Build history of the part. All positions in model axes, mm. Give positions to 0.01 mm unless a question says otherwise; leave off trailing zeros. Loops run counter-clockwise (first coordinate to the right, second up) from the corner with the lowest first, then second, coordinate; pieces in that order, holes last. Notation, with made-up numbers: (-3, 17.5) -> (49, 17.5) arc R14 ccw to (49, 34.5) -> close; hole circle Ø4 at (-36, 63). An arc over 180 degrees is marked (long way). Answer in a Markdown table with one row per item. Add a question column.
from build123d import *

# Parameters (mm, degrees)
SKETCH1_W           = 13
SKETCH1_H           = 39
BOSS_EXTRUDE1_DEPTH = 1
SKETCH2_R           = 1.35
CUT_EXTRUDE1_DEPTH  = 2
FILLET1_R           = 1


with BuildPart() as part:
    # Sketch1 → Boss-Extrude1 (new body)
    with BuildSketch(Plane(origin=(0, 0, 0), x_dir=(1, 0, 0), z_dir=(0, 1, 0))):
        Rectangle(SKETCH1_W, SKETCH1_H)
    extrude(amount=BOSS_EXTRUDE1_DEPTH)

    # Sketch2 → Cut-Extrude1 (cut, through all)
    with BuildSketch(Plane(origin=(0, 1, 0), x_dir=(1, 0, 0), z_dir=(0, 1, 0))):
        with Locations((4.5, 0)):
            Circle(SKETCH2_R)
        with Locations((4.5, -17)):
            Circle(SKETCH2_R)
        with Locations((4.5, 17)):
            Circle(SKETCH2_R)
        with Locations((-4.5, 0)):
            Circle(SKETCH2_R)
        with Locations((-4.5, 17)):
            Circle(SKETCH2_R)
        with Locations((-4.5, -17)):
            Circle(SKETCH2_R)
    extrude(amount=-CUT_EXTRUDE1_DEPTH, mode=Mode.SUBTRACT)

    # Fillet1
    fillet1_edges = [part.edges().sort_by_distance(p)[0] for p in [
        (6.5, 0.5, 19.5),
        (-6.5, 0.5, 19.5),
        (-6.5, 0.5, -19.5),
        (6.5, 0.5, -19.5),
    ]]
    fillet(fillet1_edges, radius=FILLET1_R)


solid = part.part
(1) Saw through at B-B, the plane z = 0. List the corners of the cut face in (x, y).
(2) Saw through at A-A, the plane x = 4.5. List the corners of the cut face in (y, z).
(3) Saw through at C-C, the plane y = 0.75. List the corners of the cut face in (x, z), then the cut area to 3 significant figures.
(4) Flat gauge pins, fed straight in: pin 1 Ø2.5 at (x, z) = (-4.5, 0) entering from +Y; pin 2 Ø5 at (x, z) = (-0.5, 12.5) entering from -Y. Where does each tip first touch, or does it go through?
(5) Two-plate mould, pull along Z, no slides. Class faces 1 (the flat face through (0, 1, 0)), 2 (the cylindrical face through (-6.215, 0.507, -19.199)), 3 (the cylindrical face through (4.324, 0.507, 15.661)), 4 (the cylindrical face through (-4.676, 0.507, 15.661)): released by +Z, released by -Z, zero draft, split by the parting line, or undercut.
(6) Wall check: line 1 along X through (y, z) = (0.7, -17); line 2 along Z through (x, y) = (-4.5, 0.45); line 3 along Z through (x, y) = (5.5, 0.25). Give the ranges that are in metal, low to high. Write a range as from..to.
Worked answers:
| question | item | result |
|---|---|---|
| 1 | outline | (-6.5, 0) -> (-5.85, 0) -> (-5.85, 1) -> (-6.5, 1) -> close; (-3.15, 0) -> (3.15, 0) -> (3.15, 1) -> (-3.15, 1) -> close; (5.85, 0) -> (6.5, 0) -> (6.5, 1) -> (5.85, 1) -> close |
| 2 | outline | (0, -19.5) -> (1, -19.5) -> (1, -18.35) -> (0, -18.35) -> close; (0, -15.65) -> (1, -15.65) -> (1, -1.35) -> (0, -1.35) -> close; (0, 1.35) -> (1, 1.35) -> (1, 15.65) -> (0, 15.65) -> close; (0, 18.35) -> (1, 18.35) -> (1, 19.5) -> (0, 19.5) -> close |
| 3 | outline | (-6.5, -18.5) arc R1 ccw to (-5.5, -19.5) -> (5.5, -19.5) arc R1 ccw to (6.5, -18.5) -> (6.5, 18.5) arc R1 ccw to (5.5, 19.5) -> (-5.5, 19.5) arc R1 ccw to (-6.5, 18.5) -> close; hole circle Ø2.7 at (-4.5, -17); hole circle Ø2.7 at (-4.5, 0); hole circle Ø2.7 at (-4.5, 17); hole circle Ø2.7 at (4.5, -17); hole circle Ø2.7 at (4.5, 0); hole circle Ø2.7 at (4.5, 17) |
| 3 | area | 472 mm^2 |
| 4 | pin 1 | through |
| 4 | pin 2 | y = 0 |
| 5 | face 1 | zero draft |
| 5 | face 2 | released by -Z |
| 5 | face 3 | undercut |
| 5 | face 4 | undercut |
| 6 | line 1 | -6.5..-5.85, -3.15..3.15, 5.85..6.5 |
| 6 | line 2 | -19.5..-18.35, -15.65..-1.35, 1.35..15.65, 18.35..19.5 |
| 6 | line 3 | -19.5..-17.91, -16.09..-0.91, 0.91..16.09, 17.91..19.5 |
